Design review of the part built by this model. Coordinates are the model's own, in mm. A direction names the side the tool comes from. Coordinates: 2 decimals unless noted, no trailing zeros. Loops run counter-clockwise (first coordinate to the right, second up) from the corner with the lowest first, then second, coordinate; pieces in that order, holes last. Notation, with made-up numbers: (7.25, -10.75) -> (47.25, -10.75) arc R23 cw to (47.25, 23.25) -> close; hole circle Ø6 at (-2, -29.75). An arc over 180 degrees is marked (long way). Answer as a JSON object with one key per item and string values.
```python
from build123d import *

# Parameters (mm, degrees)
EXTRUDE_5_DEPTH     = 12
EXTRUDE_6_DEPTH     = 6
SKETCH_11_R         = 2
SKETCH_11_R_2       = 0.5
EXTRUDE_7_DEPTH     = 4
CUT_EXTRUDE_4_DEPTH = 3
SKETCH_15_R         = 0.5
CUT_EXTRUDE_5_DEPTH = 38.735924528


with BuildPart() as part:
    # 草图9 → 凸台-拉伸5 (new body)
    with BuildSketch(Plane.XY):
        Polygon((11, -16.590909091), (-11, -16.590909091), (-11, 1.409090909), (-16, 1.409090909), (-16, 3.909090909), (-11, 3.909090909), (-11, 5.409090909), (11, 5.409090909), (11, 3.909090909), (16, 3.909090909), (16, 1.409090909), (11, 1.409090909), align=None)
    extrude(amount=EXTRUDE_5_DEPTH)

    # 草图10 → 凸台-拉伸6 (add)
    with BuildSketch(Plane(origin=(0, 5.409090909, 0), x_dir=(-1, 0, 0), z_dir=(0, -1, 0))):
        with BuildLine():
            ThreePointArc((0.479166667, -3.554855293), (-11, -6), (0.479166667, -8.445144707))
            ThreePointArc((0.479166667, -8.445144707), (3.5, -6), (0.479166667, -3.554855293))
        make_face()
    extrude(amount=-EXTRUDE_6_DEPTH)

    # 草图11 → 凸台-拉伸7 (add)
    with BuildSketch(Plane(origin=(0, 11.409090909, 0), x_dir=(-1, 0, 0), z_dir=(0, -1, 0))):
        with Locations(Location((-5, -6, 0), (0, 0, 90))):
            Circle(SKETCH_11_R)
        with Locations(Location((-5, -6, 0), (0, 0, 90))):
            Circle(SKETCH_11_R_2, mode=Mode.SUBTRACT)
    extrude(amount=-EXTRUDE_7_DEPTH)

    # 草图13 → 切除-拉伸4 (cut)
    with BuildSketch(Plane(origin=(0, 3.909090909, 0), x_dir=(-1, 0, 0), z_dir=(0, -1, 0))):
        with BuildLine():
            Line((-14.366025404, -6.5), (-16, -6.5))
            Line((-16, -6.5), (-16, -5.5))
            Line((-16, -5.5), (-14.366025404, -5.5))
            ThreePointArc((-14.366025404, -5.5), (-12.5, -6), (-14.366025404, -6.5))
        make_face()
        with BuildLine():
            Line((14.366025404, -5.5), (16, -5.5))
            Line((16, -5.5), (16, -6.5))
            Line((16, -6.5), (14.366025404, -6.5))
            ThreePointArc((14.366025404, -6.5), (12.5, -6), (14.366025404, -5.5))
        make_face()
    extrude(amount=CUT_EXTRUDE_4_DEPTH, mode=Mode.SUBTRACT)

    # 草图15 → 切除-拉伸5 (cut, through all)
    with BuildSketch(Plane(origin=(0, 15.409090909, 0), x_dir=(1, 0, 0), z_dir=(0, 1, 0))):
        with Locations(Location((5, -6, 0), (0, 0, 90))):
            Circle(SKETCH_15_R)
    extrude(amount=-CUT_EXTRUDE_5_DEPTH, mode=Mode.SUBTRACT)


solid = part.part
```
1) Add section B-B, the plane x = -13.5. Give the boundary of the cut face in (y, z), and give its area (3 significant figures).
Completed:
{"outline": "(1.41, 0) -> (3.91, 0) -> (3.91, 5) -> (1.41, 5) -> close; (1.41, 7) -> (3.91, 7) -> (3.91, 12) -> (1.41, 12) -> close", "area": "25.0 mm²"}
2) Add section C-C, the plane y = 13.5. Give the boundary of the cut face in (x, z), and give its area (3 significant figures).
Completed:
{"outline": "circle Ø4 at (5, 6); hole circle Ø1 at (5, 6)", "area": "11.8 mm²"}
3) Add section A-A, the plane x = -1. Give the boundary of the cut face in (y, z).
Completed:
{"outline": "(-16.59, 0) -> (5.41, 0) -> (5.41, 3.5) -> (11.41, 3.5) -> (11.41, 8.5) -> (5.41, 8.5) -> (5.41, 12) -> (-16.59, 12) -> close"}
4) Add section D-D, the plane z = 10.25. Give the boundary of the cut face in (x, y).
Completed:
{"outline": "(-16, 1.41) -> (-11, 1.41) -> (-11, -16.59) -> (11, -16.59) -> (11, 1.41) -> (16, 1.41) -> (16, 3.91) -> (11, 3.91) -> (11, 5.41) -> (9.24, 5.41) -> (9.24, 11.41) -> (0.76, 11.41) -> (0.76, 5.41) -> (-11, 5.41) -> (-11, 3.91) -> (-16, 3.91) -> close"}
5) Clearance check with flat-ended pins moving along their axes: pin 1 Ø2.5 at (x, z) = (-14.5, 8) entering from +Y; pin 2 Ø2.5 at (x, z) = (-13.5, 6) entering from -Y; pin 3 Ø2 at (y, z) = (-8, 1.5) entering from +X. State where each tip first meets the part, or that it passes through.
Completed:
{"pin 1": "y = 3.91", "pin 2": "y = 1.41", "pin 3": "x = 11"}
6) The part is to be moulded in two halves that separate along X. For faces 6 (the cylindrical face through (4.504, -0.367, 6.065)), 7 (the flat face through (-11, 5, 6)), 8 (the flat face through (11, -7, 6)), say which applies: pulls with the +X half, pulls with the -X half, needs draft (parallel to the pull), parting line crosses it, or undercut.
Completed:
{"face 6": "undercut", "face 7": "pulls with the -X half", "face 8": "pulls with the +X half"}
7) Wall thickness on probe 1 along Z at (x, y) = (5, -6.5); probe 2 along X at (y, z) = (3.2, 6); probe 3 along Z at (x, y) = (-13.5, 3.05): over which ranges is each line inside the solid? List them lowest first.
Completed:
{"probe 1": "0 to 5.5, 6.5 to 12", "probe 2": "-12.5 to 4.5, 5.5 to 12.5", "probe 3": "0 to 5, 7 to 12"}
8) For faces 1 (the flat face through (-15, 3, 5.5)), 2 (the cylindrical face through (11, 8, 6)), 3 (the flat face through (12, 3.909, 6)), 4 (the flat face through (10, 5.409, 11)), 5 (the flat face through (12, 1.409, 6)), list the 3-axis set-ups (+Z, -Z, +X, -X, +Y, -Y) from which the entire face can be reached by the end or side of a thin tool; tool diameter is ignored.
Completed:
{"face 1": "-X, +Y, -Y", "face 2": "+Y", "face 3": "+Z, -Z, +X, +Y", "face 4": "+Z, +X, +Y", "face 5": "+Z, -Z, +X, -Y"}
